Geometry check sheet. Reference: the model listing, model coordinates, mm. Give positions to 0.01 mm unless a question says otherwise; leave off trailing zeros. Write each loop counter-clockwise with the first axis right and the second up, starting at its lowest first coordinate (ties: lowest second). Pieces come first, ordered by that corner, then holes. Notation, with made-up numbers: M 69.25,74 L 111.25,74 A16 ccw 111.25,82 Z; hole C 82,-30.5 d2. An arc over 180 degrees is marked long. Write each question's results on one line, items separated by ' | '.
```python
from build123d import *

# Parameters (mm, degrees)
F0_W        = 120
F0_H        = 60
F0_W_2      = 8
F0_H_2      = 40
F1_DEPTH    = 8
F2_T1_DEPTH = 8
F2_T3_DEPTH = 9.6994572863


# Not quite as in the source:
# - a fillet or chamfer that OpenCascade refuses, or shapes differently, is made with other operations: its cross-section is extruded or revolved along the edge and cut away or added


with BuildPart() as f1:
    # F0 (on Front) → F1 (new body)
    with BuildSketch(Plane.XZ):
        with Locations((-60, -30)):
            Rectangle(F0_W, F0_H)
        with Locations((-99, -30)):
            Rectangle(F0_W_2, F0_H_2, mode=Mode.SUBTRACT)
        with Locations((-21, -30)):
            Rectangle(F0_W_2, F0_H_2, mode=Mode.SUBTRACT)
        with BuildLine():
            Line((76.0396039604, 7.603960396), (0, 0))
            Line((0, 0), (0, -60))
            Line((0, -60), (80, -32))
            ThreePointArc((80, -32), (60.0992561958, -13.9900743804), (76.0396039604, 7.603960396))
        make_face()
        with BuildLine():
            Line((-120, -60), (-120, 0))
            Line((-120, 0), (-196.0396039604, 7.603960396))
            ThreePointArc((-196.0396039604, 7.603960396), (-184.5208540159, 0.6647558051), (-180, -12))
            ThreePointArc((-180, -12), (-185.8578643763, -26.1421356237), (-200, -32))
            Line((-200, -32), (-120, -60))
        make_face()
        with BuildLine():
            ThreePointArc((80, 8), (78.0099256196, 7.9007438042), (76.0396039604, 7.603960396))
            Line((76.0396039604, 7.603960396), (80, 8))
        make_face()
        with BuildLine():
            Line((80, 8), (76.0396039604, 7.603960396))
            ThreePointArc((76.0396039604, 7.603960396), (60.0992561958, -13.9900743804), (80, -32))
            Line((80, -32), (80, -24.5))
            ThreePointArc((80, -24.5), (74.3431457505, -22.1568542495), (72, -16.5))
            Line((72, -16.5), (72, -7.5))
            ThreePointArc((72, -7.5), (74.3431457505, -1.8431457505), (80, 0.5))
            Line((80, 0.5), (80, 8))
        make_face()
        with BuildLine():
            ThreePointArc((-180, -12), (-184.5208540159, 0.6647558051), (-196.0396039604, 7.603960396))
            Line((-196.0396039604, 7.603960396), (-200, 8))
            Line((-200, 8), (-200, 0.5))
            ThreePointArc((-200, 0.5), (-194.3431457505, -1.8431457505), (-192, -7.5))
            Line((-192, -7.5), (-192, -16.5))
            ThreePointArc((-192, -16.5), (-194.3431457505, -22.1568542495), (-200, -24.5))
            Line((-200, -24.5), (-200, -32))
            ThreePointArc((-200, -32), (-185.8578643763, -26.1421356237), (-180, -12))
        make_face()
        with BuildLine():
            Line((-200, 8), (-196.0396039604, 7.603960396))
            ThreePointArc((-196.0396039604, 7.603960396), (-198.0099256196, 7.9007438042), (-200, 8))
        make_face()
        with BuildLine():
            Line((80, -24.5), (80, -32))
            ThreePointArc((80, -32), (94.1421356237, -26.1421356237), (100, -12))
            ThreePointArc((100, -12), (94.1421356237, 2.1421356237), (80, 8))
            Line((80, 8), (80, 0.5))
            ThreePointArc((80, 0.5), (85.6568542495, -1.8431457505), (88, -7.5))
            Line((88, -7.5), (88, -16.5))
            ThreePointArc((88, -16.5), (85.6568542495, -22.1568542495), (80, -24.5))
        make_face()
        with BuildLine():
            ThreePointArc((-200, 8), (-220, -12), (-200, -32))
            Line((-200, -32), (-200, -24.5))
            ThreePointArc((-200, -24.5), (-205.6568542495, -22.1568542495), (-208, -16.5))
            Line((-208, -16.5), (-208, -7.5))
            ThreePointArc((-208, -7.5), (-205.6568542495, -1.8431457505), (-200, 0.5))
            Line((-200, 0.5), (-200, 8))
        make_face()
    extrude(amount=F1_DEPTH)

    # F2: fillet of radius 2 on 7 edges, made by hand

    # F2_s2 → F2_t1 (join)
    with BuildSketch(Plane.XZ):
        with BuildLine():
            ThreePointArc((-119.9002487578, 0), (-119.9998761615, 0.0024829462), (-120.0992561958, 0.0099256196))
            Line((-120.0992561958, 0.0099256196), (-120, 0))
            Line((-120, 0), (-119.9002487578, 0))
        make_face()
        with BuildLine():
            ThreePointArc((-0.0997512422, 0), (-0.0001238385, 0.0024829462), (0.0992561958, 0.0099256196))
            Line((0.0992561958, 0.0099256196), (0, 0))
            Line((0, 0), (-0.0997512422, 0))
        make_face()
        with BuildLine():
            ThreePointArc((-200.316131174, -31.9975013709), (-199.9970841579, -32.0282320894), (-199.687043442, -32.1095347953))
            Line((-199.687043442, -32.1095347953), (-200, -32))
            ThreePointArc((-200, -32), (-200.1580705241, -31.999375333), (-200.316131174, -31.9975013709))
        make_face()
        with BuildLine():
            ThreePointArc((79.687043442, -32.1095347953), (79.997084158, -32.0282320894), (80.316131174, -31.9975013709))
            ThreePointArc((80.316131174, -31.9975013709), (80.1580705241, -31.999375333), (80, -32))
            Line((80, -32), (79.687043442, -32.1095347953))
        make_face()
        with BuildLine():
            ThreePointArc((76.1306459256, 7.6221328873), (76.0370129468, 7.6059696483), (75.9427179562, 7.5942717956))
            Line((75.9427179562, 7.5942717956), (76.0396039604, 7.603960396))
            ThreePointArc((76.0396039604, 7.603960396), (76.0851143987, 7.6130994677), (76.1306459256, 7.6221328873))
        make_face()
        with BuildLine():
            ThreePointArc((-195.9427179562, 7.5942717956), (-196.0370129468, 7.6059696483), (-196.1306459256, 7.6221328873))
            ThreePointArc((-196.1306459256, 7.6221328873), (-196.0851143987, 7.6130994677), (-196.0396039604, 7.603960396))
            Line((-196.0396039604, 7.603960396), (-195.9427179562, 7.5942717956))
        make_face()
    extrude(amount=F2_T1_DEPTH)

    # F2_s4 → F2_t3 (cut)
    with BuildSketch(Plane.XZ.offset(-0.8497286432)):
        with BuildLine():
            ThreePointArc((-120.3208093922, -59.8877167127), (-119.9951955274, -59.9717293711), (-119.6601085427, -60))
            Line((-119.6601085427, -60), (-120, -60))
            Line((-120, -60), (-120.3208093922, -59.8877167127))
        make_face()
    extrude(amount=F2_T3_DEPTH, mode=Mode.SUBTRACT)


solid = f1.part
```
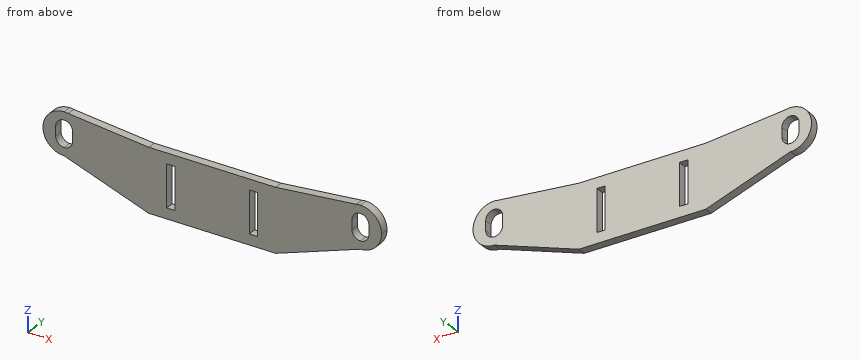
Q1. Material ranges on probe 1 along X at (y, z) = (-3.5, -27); probe 2 along X at (y, z) = (-2.5, -14); probe 3 along Z at (x, y) = (-67.5, -4), recorded low to high. Write a range as [from, to].
Answer key:
probe 1: x = [-213.23, -103], [-95, -25], [-17, 93.23] | probe 2: x = [-219.9, -208], [-192, -103], [-95, -25], [-17, 72], [88, 99.9] | probe 3: z = [-60, 0]
Q2. Section check B-B (z = -54.5). Enter the section's corners in (x, y), then the cut area to 3 significant figures.
Answer key:
outline: M -135.71,-8 L 15.71,-8 L 15.71,0 L -135.71,0 Z | area: 1,210 mm2
Q3. Section check C-C (x = -160.5). Enter the section's corners in (y, z) (3 decimals), then the cut area to 3 significant figures.
Answer key:
outline: M -8,-45.825 L 0,-45.825 L 0,4.05 L -8,4.05 Z | area: 399 mm2
Q4. Section check A-A (y = -3). State how many separate pieces and enclosed holes the cut face has, then the cut area to 3 significant figures.
Answer key:
separate pieces: 1 | enclosed holes: 4 | area: 15,100 mm2
Q5. Depth check by flat-ended pin: P1, Ø1, axis at y = -5, z = -3, coming from the -X side; P2, Ø4, axis at y = -6, z = -25, coming from the +X side; P3, Ø10, axis at x = 67, z = -42, coming from the +Y side; P4, Ø3, axis at x = -85.5, y = -2, coming from the +Z side. Enter the tip coordinate at first touch or a pass-through.
Answer key:
P1: stops at x = -218.1 | P2: stops at x = 96.7 | P3: passes through | P4: stops at z = 0
